Here's how the part is built. I have some questions about the finished solid (model axes, mm). Face numbers are marked on the shaded views. A direction names the side the tool comes from. Round coordinates to 2 decimals unless told otherwise and drop trailing zeros. Write each loop counter-clockwise with the first axis right and the second up, starting at its lowest first coordinate (ties: lowest second). Pieces come first, ordered by that corner, then holes. Notation, with made-up numbers: (10.25, 17.5) - (26.25, 17.5) arc R28 cw to (26.25, 48.5) - close; hole circle Ø2 at (4, -35). An arc over 180 degrees is marked (long way). One line per item, written item: value. Start each with the question number.
Item 1: For the marked faces 4 and 5, which set-ups out of +Z, -Z, +X, -X, +Y, -Y let a thin tool reach every point of the face, with its end or its side?
Item 2: Imagine slicing it at D-D, the plane y = 67.5. Please give me the cut outline in (x, z), then the cut area to 3 significant figures.
Item 3: For P1, Ø24, axis at x = 0, z = 0, coming from the +Y side; P2, Ø3, axis at x = 31, z = -37.5, coming from the +Y side; P3, Ø3, axis at y = 82, z = 19, coming from the -X side, each with a flat end and sliding along its axis, tell me the tip position at first contact or that it passes through.
Item 4: Thinking about a two-plate mould opening in Z: for the marked faces 1, 2 and 3, which applies, released by +Z, released by -Z, zero draft, split by the parting line, or undercut?
Item 5: Imagine slicing it at C-C, the plane y = 39. Please give me the cut outline in (x, z).
Item 6: Imagine slicing it at B-B, the plane z = 0. Please give me the cut outline in (x, y).
Item 7: Imagine slicing it at A-A, the plane x = 0. Please give me the cut outline in (y, z), then the cut area to 3 significant figures.
Item 8: If I drill on line 1 (Z direction, x = 0, y = 78); line 2 (Z direction, x = 38.5, y = 16); line 3 (Y direction, x = 40, z = 41), over which ranges is the centre line in solid material (lowest first)?
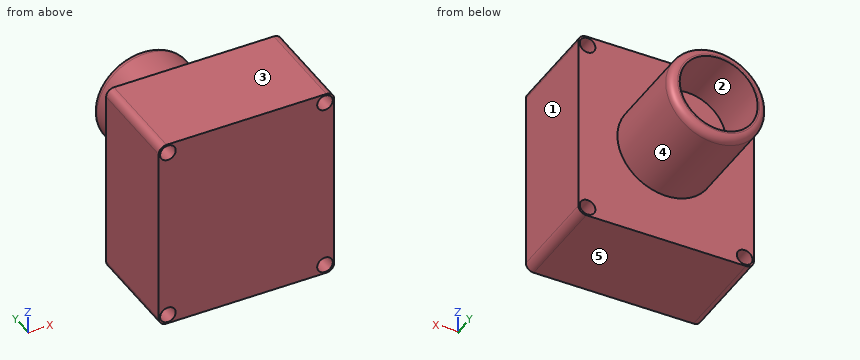
Autodesk Inventor part; units mm, degrees
ref_plane "YZ Plane" through (0, 0, 0) normal (1, 0, 0) x (0, 1, 0)
ref_plane "XZ Plane" through (0, 0, 0) normal (0, 1, 0) x (-1, 0, 0)
ref_plane "XY Plane" through (0, 0, 0) normal (0, 0, 1) x (1, 0, 0)
sketch "Boceto1" plane through (0, 0, 0) normal (0, 1, 0) x (-1, 0, 0)
  line L0 (41, 50) -> (-41, 50)
  line L1 (-45, 46) -> (-45, -46)
  line L2 (-41, -50) -> (41, -50)
  line L3 (45, -46) -> (45, 46)
  line L4 (45, 50) -> (-45, -50) construction
  line L5 (-45, 50) -> (45, -50) construction
  arc A0 (45, 46) -> (41, 50) centre (41, 46) ccw
  arc A1 (41, -50) -> (45, -46) centre (41, -46) ccw
  arc A2 (-41, 50) -> (-45, 46) centre (-41, 46) ccw
  arc A3 (-45, -46) -> (-41, -50) centre (-41, -46) ccw
  line L6 (43.8284, -48.8284) -> (40.2929, -45.2929)
  line L7 (-43.8284, -48.8284) -> (-40.2929, -45.2929)
  line L8 (-43.8284, 48.8284) -> (-40.2929, 45.2929)
  circle A4 centre (-40.2929, 45.2929) radius 4
  line L9 (43.8284, 48.8284) -> (40.2929, 45.2929)
  circle A5 centre (40.2929, 45.2929) radius 4
  circle A6 centre (40.2929, -45.2929) radius 4
  circle A7 centre (-40.2929, -45.2929) radius 4
  point P0 (0, 0)
  dimension "d1" = 90
  dimension "d2" = 100
  dimension "d3" = 4
  dimension "d5" = 5
  dimension "d6" = 5
  dimension "d7" = 5
  dimension "d9" = 8
  dimension "d10" = 5
  dimension "d11" = 8
  dimension "d12" = 8
  dimension "d13" = 8
extrude "Extrusión1" add sketch "Boceto1" along normal blind 50
sketch "Boceto2" plane through (0, 50, 0) normal (0, 1, 0) x (1, 0, 0)
  circle A0 centre (0, 0) radius 25
  dimension "d16" = 50
extrude "Extrusión2" add sketch "Boceto2" along normal blind 50
sketch "Boceto3" plane through (0, 100, 0) normal (0, 1, 0) x (1, 0, 0)
  circle A0 centre (0, 0) radius 20
  dimension "d19" = 40
extrude "Extrusión3" cut sketch "Boceto3" against normal blind 30
thread "Rosca1"
fillet "Empalme1" radius 4 1 edges at (-25, 100, 0)
properties part number "Tarea 01 Ayala Dinamica"
Values follow:
1. face 4: +Y
1. face 5: -Z, +X, -X, +Y, -Y
2. outline: circle Ø50 at (0, 0)
2. area: 1,960 mm^2
3. P1: stops at y = 70
3. P2: stops at y = 50
3. P3: stops at x = -17.85
4. face 1: zero draft
4. face 2: undercut
4. face 3: released by +Z
5. outline: (-45, -46) arc R4 ccw to (-41, -50) - (41, -50) arc R4 ccw to (45, -46) - (45, 46) arc R4 ccw to (41, 50) - (-41, 50) arc R4 ccw to (-45, 46) - close; hole circle Ø8 at (-40.29, -45.29); hole circle Ø8 at (-40.29, 45.29); hole circle Ø8 at (40.29, -45.29); hole circle Ø8 at (40.29, 45.29)
6. outline: (-45, 0) - (45, 0) - (45, 50) - (25, 50) - (25, 96) arc R4 ccw to (21, 100) - (20, 100) - (20, 70) - (-20, 70) - (-20, 100) - (-21, 100) arc R4 ccw to (-25, 96) - (-25, 50) - (-45, 50) - close
7. outline: (0, -50) - (50, -50) - (50, -25) - (96, -25) arc R4 ccw to (100, -21) - (100, -20) - (70, -20) - (70, 20) - (100, 20) - (100, 21) arc R4 ccw to (96, 25) - (50, 25) - (50, 50) - (0, 50) - close
7. area: 6,290 mm^2
8. line 1: z = -25 to -20, 20 to 25
8. line 2: z = -50 to -48.87, -41.72 to 41.72, 48.87 to 50
8. line 3: y = 0 to 50
